Geometry: final body of the model. Coordinates: model frame, mm. Face numbers are marked on the shaded views. A direction names the side the tool comes from. Give positions to 0.01 mm unless a question says otherwise; leave off trailing zeros. Loops run counter-clockwise (first coordinate to the right, second up) from the corner with the lowest first, then second, coordinate; pieces in that order, holes last.
1. Access query for the marked faces 1, 2 and 3. Directions: +Z, -Z, +X, -X, +Y, -Y. A direction counts if a zero-diameter tool reaches every point of the face in a straight line with its end or side. Return the directions, or none.
2. First-contact query: P1, Ø9, axis at x = 5, z = -9.5, coming from the +Y side; P2, Ø9, axis at x = 5.5, z = -6.5, coming from the -Y side; P3, Ø0.8, axis at x = 10.5, y = -1.5, coming from the +Z side. Flat tips, straight axial feed; report the tip coordinate or a pass-through.
3. Material intervals for line 1 along Y through (x, z) = (6, -13.5); line 2 along Z through (x, y) = (2.5, -0.5); line 3 along Z through (x, y) = (9.5, 2.75), sorted ascending.
4. Section B-B, the plane z = -19.75. Output: boundary loops of the cut face in (x, y), then the cut area to 3 significant figures.
5. Section C-C, the plane y = -2. Output: boundary loops of the cut face in (x, z).
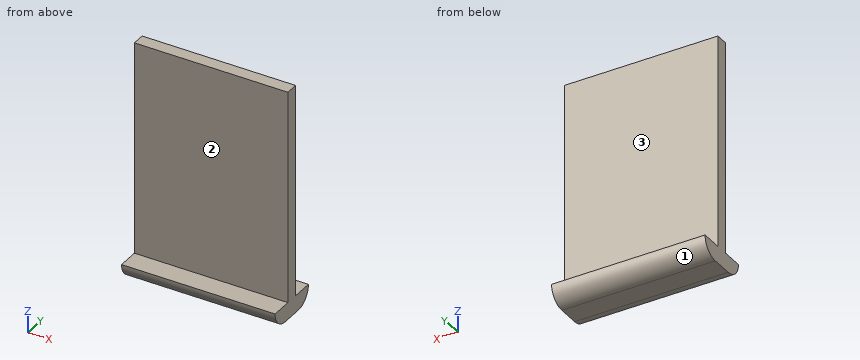
from build123d import *

# Parameters (mm, degrees)
SKETCH1_W           = 18
SKETCH1_H           = 25
BOSS_EXTRUDE1_DEPTH = 1.5
BOSS_EXTRUDE2_DEPTH = 2
FILLET1_R           = 2


with BuildPart() as part:
    # Sketch1 → Boss-Extrude1 (new body)
    with BuildSketch(Plane(origin=(0, 0, 0), x_dir=(1, 0, 0), z_dir=(0, 1, 0))):
        with Locations((9, 12.5)):
            Rectangle(SKETCH1_W, SKETCH1_H)
    extrude(amount=BOSS_EXTRUDE1_DEPTH)

    # Sketch2 → Boss-Extrude2 (add)
    with BuildSketch(Plane(origin=(0, 0, -25), x_dir=(-1, 0, 0), z_dir=(0, 0, -1))):
        Polygon((-18, 0), (-18, -2.5), (0, -2.5), (0, 4), (-18, 4), align=None)
    extrude(amount=BOSS_EXTRUDE2_DEPTH)

    # Fillet1
    fillet1_edges = [part.edges().sort_by_distance(p)[0] for p in [
        (9, 4, -27),
        (9, -2.5, -27),
    ]]
    fillet(fillet1_edges, radius=FILLET1_R - 0.0001)  # a hair under: the kernel refuses the full size


solid = part.part
Answers below:
1. face 1: -Z, +X, -X, +Y
1. face 2: +Z, +X, -X, -Y
1. face 3: +Z, +X, -X, +Y
2. P1: stops at y = 1.5
2. P2: stops at y = 0
2. P3: stops at z = -25
3. line 1: y = 0 to 1.5
3. line 2: z = -27 to -25
3. line 3: z = -26.85 to -25
4. outline: (0, 0) - (18, 0) - (18, 1.5) - (0, 1.5) - close
4. area: 27.0 mm2
5. outline: (0, -26.32) - (18, -26.32) - (18, -25) - (0, -25) - close
